Verification items for this drawing (mm, ordinates from the low corner). Round coordinates to 2 decimals unless told otherwise and drop trailing zeros. Loops run counter-clockwise (first coordinate to the right, second up) from the corner with the lowest first, then second, coordinate; pieces in that order, holes last. Notation, with made-up numbers: M -5,-25 L 52,-25 A23 ccw 52,0 Z; hole C -1,-12.75 d3. An arc over 180 degrees is marked long. Write item = value, one per line.
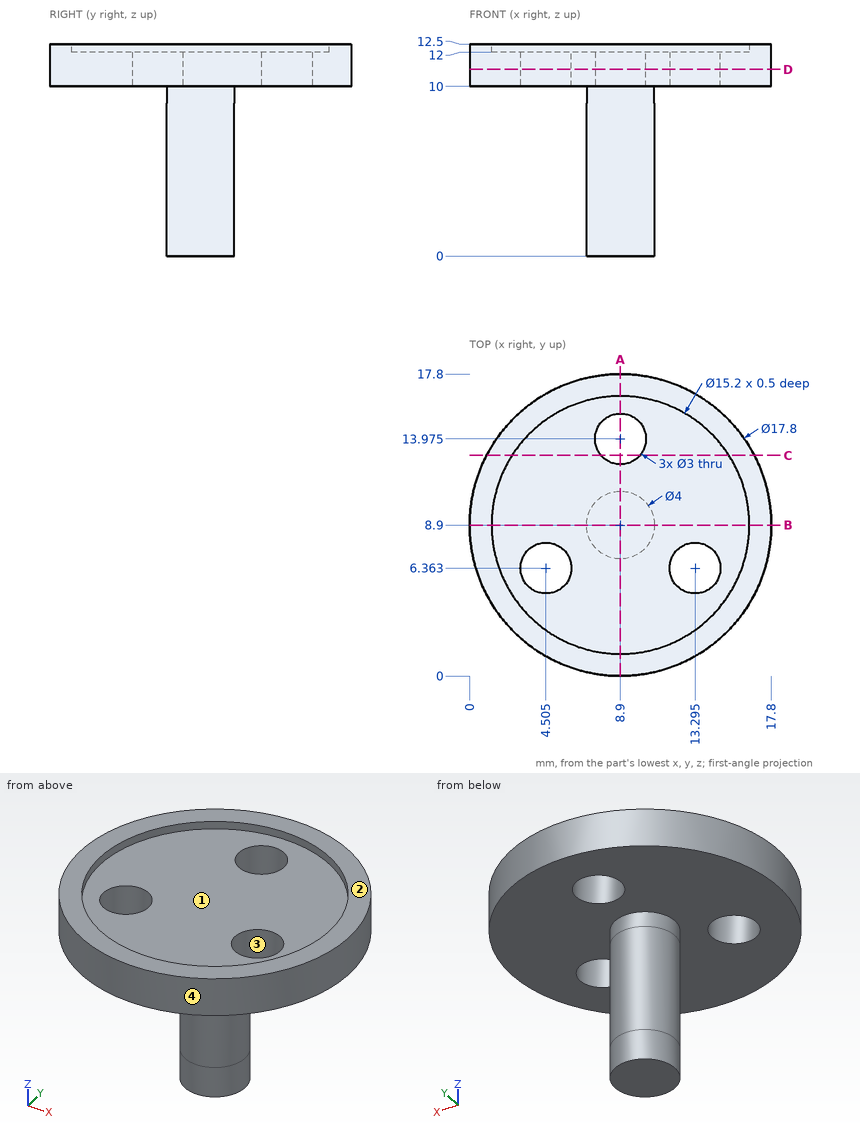
(1) Sectioned sample at D-D on z = 11. Record the cut outline in (x, y) (1 decimal).
Result set:
outline = C 8.9,8.9 d17.8; hole C 4.5,6.4 d3; hole C 8.9,14 d3; hole C 13.3,6.4 d3
(2) Sectioned sample at A-A on x = 8.9. Record the cut outline in (y, z) (1 decimal).
Result set:
outline = M 0,10 L 6.9,10 L 6.9,0 L 10.9,0 L 10.9,10 L 12.5,10 L 12.5,12 L 1.3,12 L 1.3,12.5 L 0,12.5 Z; M 15.5,10 L 17.8,10 L 17.8,12.5 L 16.5,12.5 L 16.5,12 L 15.5,12 Z
(3) Depth check by flat-ended pin: pin 1 Ø1 at (y, z) = (8, 7.5) entering from -X; pin 2 Ø1.8 at (x, y) = (13.3, 6.36) entering from +Z; pin 3 Ø4.5 at (x, y) = (10, 6) entering from +Z; pin 4 Ø6 at (y, z) = (3.5, 10.5) entering from +X. Enter the tip coordinate at first touch or a pass-through.
Result set:
pin_1 = 6.94
pin_2 = through
pin_3 = 12
pin_4 = 17.47
(4) Sectioned sample at B-B on y = 8.9. Record the cut outline in (x, z).
Result set:
outline = M 0,10 L 6.9,10 L 6.9,0 L 10.9,0 L 10.9,10 L 17.8,10 L 17.8,12.5 L 16.5,12.5 L 16.5,12 L 1.3,12 L 1.3,12.5 L 0,12.5 Z
(5) Release check for a two-part mould opening along X. For the marked faces 1, 2, 3 and 4 record: released by +X, released by -X, zero draft, split by the parting line, or undercut.
Result set:
face_1 = undercut
face_2 = zero draft
face_3 = undercut
face_4 = split by the parting line
(6) Sectioned sample at C-C on y = 13. Record the cut outline in (x, z).
Result set:
outline = M 1,10 L 7.76,10 L 7.76,12 L 2.5,12 L 2.5,12.5 L 1,12.5 Z; M 10.04,10 L 16.8,10 L 16.8,12.5 L 15.3,12.5 L 15.3,12 L 10.04,12 Z
(7) Material ranges on line 1 along Y through (x, z) = (8.9, 12.25); line 2 along Y through (x, z) = (8.9, 11) (1 decimal); line 3 along Z through (x, y) = (10, 3.25), recorded low to high. Write a range as from..to.
Result set:
line_1 = 0..1.3, 16.5..17.8
line_2 = 0..12.5, 15.5..17.8
line_3 = 10..12
